The listing builds one solid part. Answer for the finished solid, in the listing's coordinates (mm). A direction names the side the tool comes from. Coordinates: 2 decimals unless noted, no trailing zeros. Order: outer loops, then holes, each group sorted by start corner. A loop starts at its lowest first (then second) coordinate and runs counter-clockwise, first axis right, second up. Notation, with made-up numbers: (40.5, -17) -> (97.5, -17) arc R28 cw to (97.5, 14) -> close; hole circle Ø3 at (62.5, 20). An arc over 180 degrees is marked (long way). Answer in a Markdown table with one row per item. Add a question column.
```python
from build123d import *

# Parameters (mm, degrees)
BOSS_EXTRUDE1_DEPTH             = 6.35
CUT_EXTRUDE1_DEPTH              = 56.448991199
CUT_EXTRUDE2_DEPTH              = 56.448991199
FILLET1_R                       = 6.858
F_6_0MM_CLEARANCE_DOWEL_HOLE1_D = 6
FILLET2_R                       = 0.508


with BuildPart() as part:
    # Sketch1 → Boss-Extrude1 (new, symmetric)
    with BuildSketch(Plane.XY):
        Polygon((-47.625, 0), (47.625, 0), (47.625, 9.525), (31.75, 25.4), (-31.75, 25.4), (-47.625, 9.525), align=None)
    extrude(amount=BOSS_EXTRUDE1_DEPTH, both=True)

    # Sketch2 → Cut-Extrude1 (cut, through all)
    with BuildSketch(Plane.XY.offset(6.35)):
        with BuildLine():
            Line((-34.8361, 9.525), (-34.8361, 4.7625))
            ThreePointArc((-34.8361, 4.7625), (-38.1, 1.4986), (-41.3639, 4.7625))
            Line((-41.3639, 4.7625), (-41.3639, 9.525))
            ThreePointArc((-41.3639, 9.525), (-38.1, 12.7889), (-34.8361, 9.525))
        make_face()
        with BuildLine():
            Line((41.3639, 9.525), (41.3639, 4.7625))
            ThreePointArc((41.3639, 4.7625), (38.1, 1.4986), (34.8361, 4.7625))
            Line((34.8361, 4.7625), (34.8361, 9.525))
            ThreePointArc((34.8361, 9.525), (38.1, 12.7889), (41.3639, 9.525))
        make_face()
    extrude(amount=-CUT_EXTRUDE1_DEPTH, mode=Mode.SUBTRACT)

    # Sketch3 → Cut-Extrude2 (cut, through all)
    with BuildSketch(Plane.XY.offset(6.35)):
        Polygon((-30.574434976, 4.018858704), (-19.349114825, 15.244178855), (19.349114825, 15.244178855), (30.574434976, 4.018858704), (30.574434976, 0), (-30.574434976, 0), align=None)
    extrude(amount=-CUT_EXTRUDE2_DEPTH, mode=Mode.SUBTRACT)

    # Fillet1
    fillet1_edges = [part.edges().sort_by_distance(p)[0] for p in [
        (-19.349114825, 15.244178855, 0),
        (19.349114825, 15.244178855, 0),
        (30.574434976, 4.018858704, 0),
        (-30.574434976, 4.018858704, 0),
    ]]
    fillet(fillet1_edges, radius=FILLET1_R)

    # Ø6.0mm Clearance Dowel Hole1 (through all)
    with Locations(Plane(origin=(-17.29664684, 17.29664684, 0), x_dir=(-0.7071067811865511, -0.7071067811865439, 0), z_dir=(0.7071067811865439, -0.7071067811865511, 0))):
        with Locations((10.840128061, 0)):
            f_6_0mm_clearance_dowel_hole1 = Hole(F_6_0MM_CLEARANCE_DOWEL_HOLE1_D / 2)

    # Mirror2: Ø6.0mm Clearance Dowel Hole1 across plane
    add(f_6_0mm_clearance_dowel_hole1.mirror(Plane(origin=(0, 0, 0), x_dir=(0, 0, 1), z_dir=(1, 0, 0))), mode=Mode.SUBTRACT)

    # Fillet2
    fillet2_edges = [part.edges().sort_by_distance(p)[0] for p in [
        (-47.625, 9.525, 0),
        (-31.75, 25.4, 0),
        (31.75, 25.4, 0),
        (47.625, 9.525, 0),
        (47.625, 0, 0),
        (-47.625, 0, 0),
        (30.574434976, 0, 0),
        (-30.574434976, 0, 0),
    ]]
    fillet(fillet2_edges, radius=FILLET2_R)


solid = part.part
```
Q1. A cutting plane is placed at A-A (y = 2.5). Determine the outline of the cut face in (x, z) (3 decimals).
Q2. A cutting plane is placed at C-C (x = -9). Determine the outline of the cut face in (y, z).
Q3. For faces 5 (the face through (-38.17, 12.79, 0.09)), 6 (the face through (30.067, 3.768, -0.089)), 7 (the face through (-39, 0, 0)), determine the directions among +Z, -Z, +X, -X, +Y, -Y from which every point of the face is accessible in a straight line to the end or side of a thin tool.
Q4. A cutting plane is placed at B-B (z = -2). State how many separate pieces and enclosed holes the cut face has, then the cut area to 3 significant figures.
Q5. Determine the mould class of faces 1 (the face through (32.36, 13.67, 1.83)), 2 (the face through (38.03, 12.79, 0.09)), 3 (the face through (-1, 16, -6.35)), 4 (the face through (-1, 16, 6.35)) for opening direction Z: +Z half, -Z half, draft (parallel to the pull), parting line (faces both ways), or undercut.
Q6. Given pin 1 (5 mm diameter, centred on y = 21, z = 1.5, fed in from -X); pin 2 (1.5 mm diameter, centred on x = -6, z = 2, fed in from -Y), each flat-ended and moving along its own axis, determine where each tip first touches the part or whether it passes through.
Q7. Straight lines are drawn through the part: line 1 (X direction, y = 6.75, z = -4) (3 decimals); line 2 (X direction, y = 3.75, z = 1.5) (3 decimals); line 3 (X direction, y = 19.25, z = -2.5). For each, find the intervals that lie inside material, in ascending order.
Returned:
| question | item | result |
|---|---|---|
| 1 | outline | (-47.625, -6.35) -> (-40.452, -6.35) -> (-40.452, 6.35) -> (-47.625, 6.35) -> close; (-35.748, -6.35) -> (-30.446, -6.35) -> (-30.446, 6.35) -> (-35.748, 6.35) -> close; (30.446, -6.35) -> (35.748, -6.35) -> (35.748, 6.35) -> (30.446, 6.35) -> close; (40.452, -6.35) -> (47.625, -6.35) -> (47.625, 6.35) -> (40.452, 6.35) -> close |
| 2 | outline | (15.24, -6.35) -> (25.4, -6.35) -> (25.4, 6.35) -> (15.24, 6.35) -> close |
| 3 | face 5 | +Z, -Z |
| 3 | face 6 | +Z, -Z, -Y |
| 3 | face 7 | +Z, -Z, +X, -X, -Y |
| 4 | separate pieces | 3 |
| 4 | enclosed holes | 2 |
| 4 | area | 1,090 mm² |
| 5 | face 1 | undercut |
| 5 | face 2 | draft |
| 5 | face 3 | -Z half |
| 5 | face 4 | +Z half |
| 6 | pin 1 | stops at x = -38.65 |
| 6 | pin 2 | stops at y = 15.24 |
| 7 | line 1 | x = -47.625 to -41.364, -34.836 to -27.843, 27.843 to 34.836, 41.364 to 47.625 |
| 7 | line 2 | x = -47.625 to -41.203, -34.997 to -30.074, 30.074 to 34.997, 41.203 to 47.625 |
| 7 | line 3 | x = -37.9 to -36.93, -32.24 to 32.24, 36.93 to 37.9 |
